Part model, mm, in its own coordinate system. Face numbers are marked on the shaded views. A direction names the side the tool comes from. Give positions to 0.01 mm unless a question says otherwise; leave off trailing zeros. Order: outer loops, then holes, each group sorted by start corner. A loop starts at its lowest first (then second) coordinate and runs counter-clockwise, first axis right, second up. Notation, with made-up numbers: (14, -29.5) -> (26, -29.5) arc R23 ccw to (26, -10.5) -> close; hole circle Ø6 at (38.25, 71.25). An arc over 180 degrees is marked (long way). Write item = value, one per line. Start each with the question number.
Item 1: Band-saw the part on D-D on y = 0.6. Count the separate pieces of the cut face and the enclosed holes in it, plus the area to 3 significant figures.
Item 2: Band-saw the part on C-C on z = 8.5. Write the cut outline in (x, y), plus the area to 3 significant figures.
Item 3: Tool access for the marked faces 1 and 2: list every direction of +Z, -Z, +X, -X, +Y, -Y with a clear straight run to the whole face (end or side of a thin tool).
Item 4: Flat gauge pins, fed straight in: P1, Ø2.5, axis at x = 24, z = 0, coming from the +Y side; P2, Ø1, axis at x = 24, y = 0.5, coming from the +Z side; P3, Ø4.5, axis at x = 13.5, z = -2.5, coming from the -Y side. Where does each tip first touch, or does it go through?
Item 5: Band-saw the part on A-A on x = 24. Write the cut outline in (y, z).
Item 6: Band-saw the part on B-B on z = 0.5. Write the cut outline in (x, y), plus the area to 3 significant figures.
Item 7: Drill centre lines: line 1 along X through (y, z) = (0.65, 0); line 2 along X through (y, z) = (1.45, -2.5); line 3 along X through (y, z) = (1.55, 3.5). Where is each one in solid material? Low to high.
```python
from build123d import *

# Parameters (mm, degrees)
SKETCH_1_W          = 62
SKETCH_1_H          = 15
SKETCH_1_R          = 1.5
SKETCH_1_R_2        = 1.1
SKETCH_1_R_3        = 4
EXTRUDE_1_DEPTH     = 2
SKETCH_2_R          = 1.4
EXTRUDE_2_DEPTH     = 2
SKETCH_3_R          = 3
CUT_EXTRUDE_1_DEPTH = 1.5


with BuildPart() as part:
    # 草图1 → 凸台-拉伸1 (new body)
    with BuildSketch(Plane(origin=(0, 0, 0), x_dir=(1, 0, 0), z_dir=(0, 1, 0))):
        Rectangle(SKETCH_1_W, SKETCH_1_H)
        with Locations(Location((-8, 0, 0), (0, 0, 270))):
            Circle(SKETCH_1_R, mode=Mode.SUBTRACT)
        with Locations(Location((-3.669872981, 2.5, 0), (0, 0, 270))):
            Circle(SKETCH_1_R_2, mode=Mode.SUBTRACT)
        with Locations(Location((-12.330127019, -2.5, 0), (0, 0, 270))):
            Circle(SKETCH_1_R_2, mode=Mode.SUBTRACT)
        with Locations(Location((8, 0, 0), (0, 0, 270))):
            Circle(SKETCH_1_R_3, mode=Mode.SUBTRACT)
        with Locations(Location((24, 0, 0), (0, 0, 270))):
            Circle(SKETCH_1_R, mode=Mode.SUBTRACT)
        with Locations(Location((27.5, 0, 0), (0, 0, 270))):
            Circle(SKETCH_1_R_2, mode=Mode.SUBTRACT)
        with Locations(Location((24, -3.5, 0), (0, 0, 270))):
            Circle(SKETCH_1_R_2, mode=Mode.SUBTRACT)
        with Locations(Location((20.5, 0, 0), (0, 0, 270))):
            Circle(SKETCH_1_R_2, mode=Mode.SUBTRACT)
        with Locations(Location((24, 3.5, 0), (0, 0, 270))):
            Circle(SKETCH_1_R_2, mode=Mode.SUBTRACT)
    extrude(amount=EXTRUDE_1_DEPTH)

    # 草图2 → 凸台-拉伸2 (add)
    with BuildSketch(Plane.XY.offset(7.5)):
        with Locations(Location((-23, 0.6, 0), (0, 0, 205.376933525))):
            Circle(SKETCH_2_R)
        with Locations(Location((-8, 0.6, 0), (0, 0, 205.376933525))):
            Circle(SKETCH_2_R)
        with Locations(Location((7, 0.6, 0), (0, 0, 205.376933525))):
            Circle(SKETCH_2_R)
    extrude(amount=EXTRUDE_2_DEPTH)

    # 草图3 → 切除-拉伸1 (cut)
    with BuildSketch(Plane.XZ):
        with Locations(Location((-8, 0, 0), (0, 0, 270))):
            Circle(SKETCH_3_R)
    extrude(amount=-CUT_EXTRUDE_1_DEPTH, mode=Mode.SUBTRACT)


solid = part.part
```
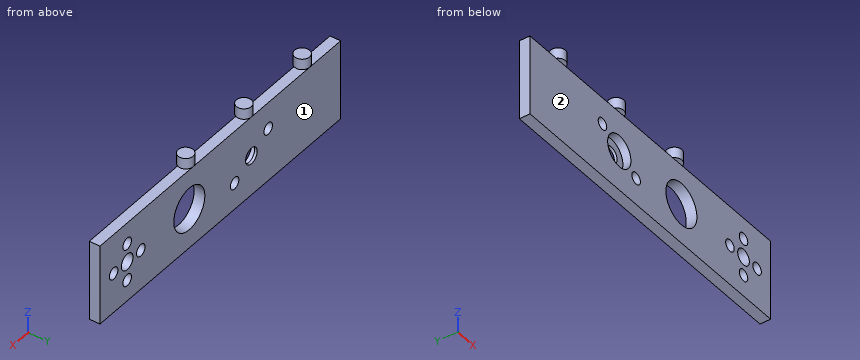
Values found:
q1.separate_pieces = 1
q1.enclosed_holes = 9
q1.area = 838 mm^2
q2.outline = circle Ø2.8 at (-23, 0.6); circle Ø2.8 at (-8, 0.6); circle Ø2.8 at (7, 0.6)
q2.area = 18.5 mm^2
q3.face_1 = +Z, -Z, +X, -X, +Y
q3.face_2 = -Z, +X, -X, -Y
q4.P1 = through
q4.P2 = 7.5
q4.P3 = 0
q5.outline = (0, -7.5) -> (2, -7.5) -> (2, -4.6) -> (0, -4.6) -> close; (0, -2.4) -> (2, -2.4) -> (2, -1.5) -> (0, -1.5) -> close; (0, 1.5) -> (2, 1.5) -> (2, 2.4) -> (0, 2.4) -> close; (0, 4.6) -> (2, 4.6) -> (2, 7.5) -> (0, 7.5) -> close
q6.outline = (-31, 0) -> (-10.96, 0) -> (-10.96, 1.5) -> (-9.41, 1.5) -> (-9.41, 2) -> (-31, 2) -> close; (-6.59, 1.5) -> (-5.04, 1.5) -> (-5.04, 0) -> (4.03, 0) -> (4.03, 2) -> (-6.59, 2) -> close; (11.97, 0) -> (19.52, 0) -> (19.52, 2) -> (11.97, 2) -> close; (21.48, 0) -> (22.59, 0) -> (22.59, 2) -> (21.48, 2) -> close; (25.41, 0) -> (26.52, 0) -> (26.52, 2) -> (25.41, 2) -> close; (28.48, 0) -> (31, 0) -> (31, 2) -> (28.48, 2) -> close
q6.area = 84.3 mm^2
q7.line_1 = -31 to -11, -5 to 4, 12 to 19.4, 21.6 to 22.5, 25.5 to 26.4, 28.6 to 31
q7.line_2 = -31 to -9.66, -6.34 to -4.77, -2.57 to 4.88, 11.12 to 23.54, 24.46 to 31
q7.line_3 = -31 to -12.79, -11.87 to 6.06, 9.94 to 22.9, 25.1 to 31
